Verification items for this drawing (mm, ordinates from the low corner). A direction names the side the tool comes from. Give positions to 0.01 mm unless a question says otherwise; leave off trailing zeros. Loops run counter-clockwise (first coordinate to the right, second up) from the corner with the lowest first, then second, coordinate; pieces in that order, holes last. Notation, with made-up numbers: (76, 13) - (93, 13) arc R19 cw to (93, 46) - close; hole circle Ø8 at (49, 42.5). An arc over 180 degrees is marked (long way). Write item = value, one per line. Start each with the question number.
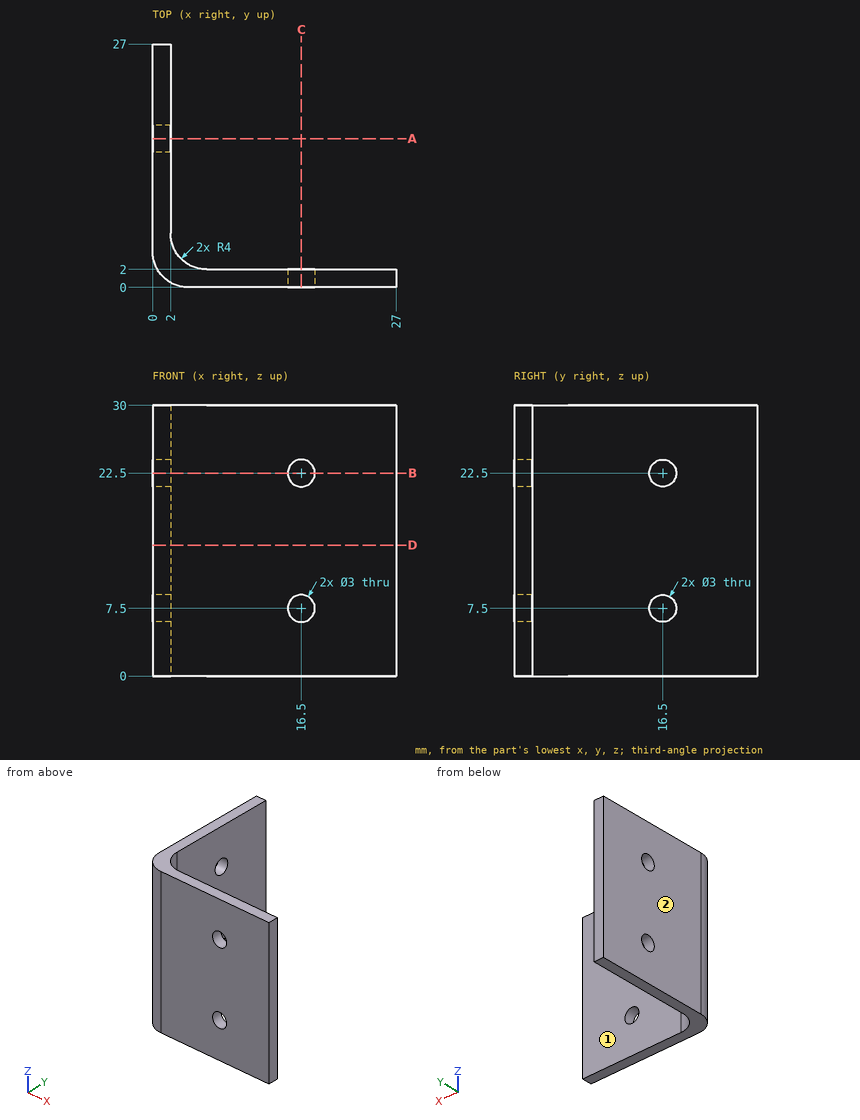
1) Cross-section at B-B on z = 22.5. Enter the section's corners in (x, y).
2) Gauge pin test, flat ends, axial feed: P1, Ø12, axis at y = 8.5, z = 18, coming from the +X side; P2, Ø5, axis at x = 16.5, z = 7.5, coming from the +Y side; P3, Ø6.5, axis at y = 16, z = 12, coming from the +X side; P4, Ø2.5, axis at y = 16.5, z = 22.5, coming from the -X side. Record the tip position at first contact, or that the pin passes through.
3) Material ranges on line 1 along Z through (x, y) = (16.5, 0.8); line 2 along Y through (x, z) = (23.5, 26.75), recorded low to high.
4) Cross-section at A-A on y = 16.5. Enter the section's corners in (x, z).
5) Cross-section at D-D on z = 14.5. Enter the section's corners in (x, y), and give its area (3 significant figures).
6) Tool access check on the marked faces 1 and 2. Record the directions out of +Z, -Z, +X, -X, +Y, -Y that give a thin tool (end or side, any length) a straight path to the whole face; none if there is none.
Checked values:
q1.outline = (0, 4) arc R4 ccw to (4, 0) - (15, 0) - (15, 2) - (6, 2) arc R4 cw to (2, 6) - (2, 15) - (0, 15) - close; (0, 18) - (2, 18) - (2, 27) - (0, 27) - close; (18, 0) - (27, 0) - (27, 2) - (18, 2) - close
q2.P1 = 4.06
q2.P2 = 2
q2.P3 = 2
q2.P4 = through
q3.line_1 = 0 to 6, 9 to 21, 24 to 30
q3.line_2 = 0 to 2
q4.outline = (0, 0) - (2, 0) - (2, 6) - (0, 6) - close; (0, 9) - (2, 9) - (2, 21) - (0, 21) - close; (0, 24) - (2, 24) - (2, 30) - (0, 30) - close
q5.outline = (0, 4) arc R4 ccw to (4, 0) - (27, 0) - (27, 2) - (6, 2) arc R4 cw to (2, 6) - (2, 27) - (0, 27) - close
q5.area = 104 mm²
q6.face_1 = +Z, -Z, +X, +Y
q6.face_2 = +Z, -Z, -X, +Y, -Y
